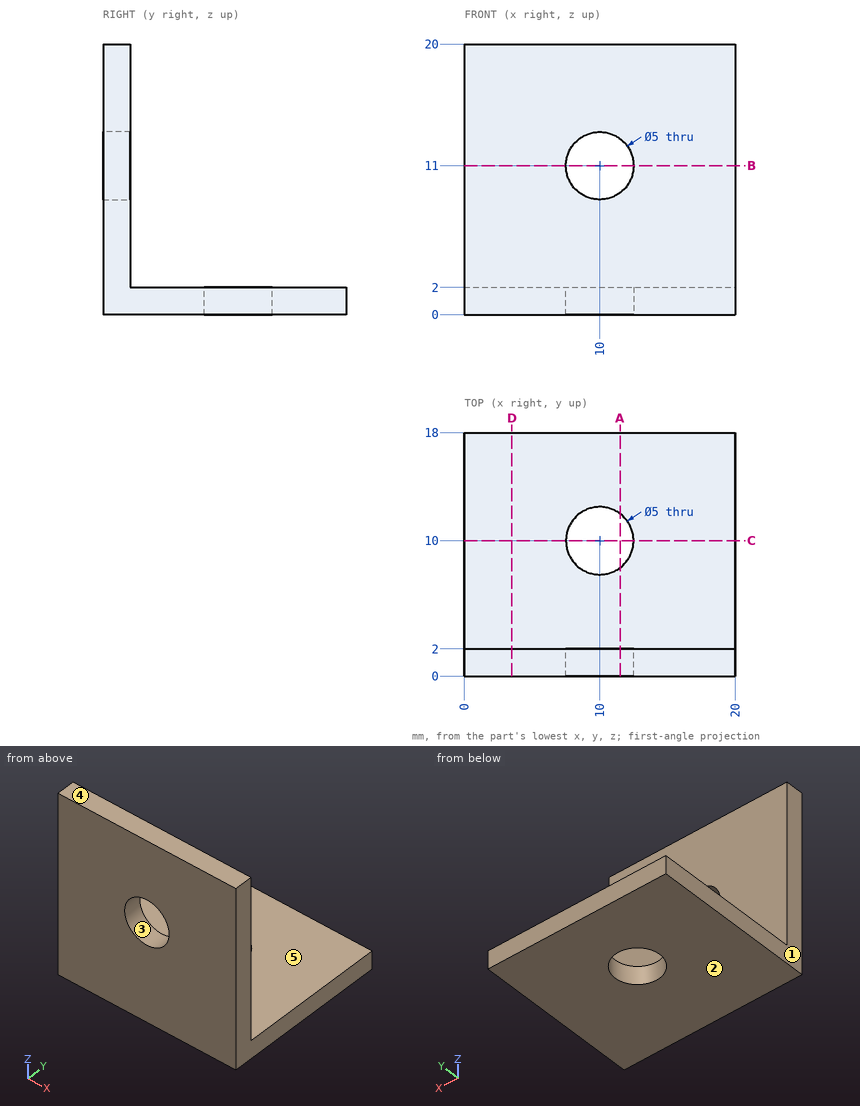
Input: dimensioned drawing with shaded views. Units: mm. Origin: part minimum x, y, z. A direction names the side the tool comes from. Coordinates: 2 decimals unless noted, no trailing zeros. Write each loop counter-clockwise with the first axis right and the second up, starting at its lowest first coordinate (ties: lowest second). Pieces come first, ordered by that corner, then holes. Notation, with made-up numbers: (-2, 24) -> (19, 24) arc R23 ccw to (19, 56) -> close; hole circle Ø11 at (59.5, 49.25). An arc over 180 degrees is marked (long way). Return JSON: item names as keys, results as strings. Group by question number.
1) Set-up query: the marked faces 4 and 5. Return all of +Z, -Z, +X, -X, +Y, -Y with unobstructed straight access to the full face (end or side cutting, diameter ignored); none if empty.
2) Section query D-D, the plane x = 3.5. Return loops of the section in (y, z), plus the area to 3 significant figures.
3) Section query B-B, the plane z = 11. Return loops of the section in (x, y), plus the area to 3 significant figures.
4) Ray query, line 1 along Y through (x, z) = (10, 1); line 2 along X through (y, z) = (0.95, 11); line 3 along Z through (x, y) = (10.5, 16.75). Return the intervals inside material, ascending.
5) Section query A-A, the plane x = 11.5. Return loops of the section in (y, z), plus the area to 3 significant figures.
6) Mould query, pull axis X, two halves, no side actions, for the marked faces 1, 2 and 3. Classes: +X half, -X half, draft (parallel to the pull), parting line (faces both ways), or undercut.
7) Contact query for flat-ended pins moving along their axis: P1, Ø4, axis at x = 10, y = 10, coming from the -Z side; P2, Ø1.5, axis at x = 7, z = 15.5, coming from the +Y side. Output: stop coordinate, or through.
From the geometry:
{
 "1": {"face 4": "+Z, +X, -X, +Y, -Y", "face 5": "+Z, +X, -X, +Y"},
 "2": {"outline": "(0, 0) -> (18, 0) -> (18, 2) -> (2, 2) -> (2, 20) -> (0, 20) -> close", "area": "72.0 mm²"},
 "3": {"outline": "(0, 0) -> (7.5, 0) -> (7.5, 2) -> (0, 2) -> close; (12.5, 0) -> (20, 0) -> (20, 2) -> (12.5, 2) -> close", "area": "30.0 mm²"},
 "4": {"line 1": "0 to 7.5, 12.5 to 18", "line 2": "0 to 7.5, 12.5 to 20", "line 3": "0 to 2"},
 "5": {"outline": "(0, 0) -> (8, 0) -> (8, 2) -> (2, 2) -> (2, 9) -> (0, 9) -> close; (0, 13) -> (2, 13) -> (2, 20) -> (0, 20) -> close; (12, 0) -> (18, 0) -> (18, 2) -> (12, 2) -> close", "area": "56.0 mm²"},
 "6": {"face 1": "-X half", "face 2": "draft", "face 3": "undercut"},
 "7": {"P1": "through", "P2": "y = 2"}
}
